from build123d import *

# Parameters (mm, degrees)
SKETCH1_W                       = 28.5
SKETCH1_H                       = 61
SKETCH1_W_2                     = 20.5
SKETCH1_H_2                     = 43
BOSS_EXTRUDE1_DEPTH             = 8
SKETCH2_W                       = 4
SKETCH2_H                       = 52
BOSS_EXTRUDE2_DEPTH             = 55
SKETCH3_W                       = 28.5
SKETCH3_H                       = 12
BOSS_EXTRUDE3_DEPTH             = 4
CUT_EXTRUDE1_DEPTH              = 93.207646104
CUT_EXTRUDE1_DEPTH_BACK         = 93.207646104
SKETCH5_W                       = 15
SKETCH5_H                       = 5.682620757
BOSS_EXTRUDE4_DEPTH             = 20.5
CUT_EXTRUDE2_DEPTH              = 93.207646104
CUT_EXTRUDE2_DEPTH_BACK         = 4
SKETCH7_W                       = 20.5
SKETCH7_H                       = 7
F_3_0MM_DOWEL_HOLE1_D           = 3
F_3_0MM_DOWEL_HOLE1_DEPTH       = 4
F_3_0MM_DOWEL_HOLE1_CSINK_D     = 3.05
F_3_0MM_DOWEL_HOLE1_CSINK_ANGLE = 100
F_3_0MM_DOWEL_HOLE1_TIP         = 0.901290929
SKETCH19_R                      = 2
CUT_EXTRUDE3_DEPTH              = 4
SKETCH21_W                      = 28.5
SKETCH21_H                      = 15
BOSS_EXTRUDE5_DEPTH             = 9
SKETCH24_R                      = 2
CUT_EXTRUDE6_DEPTH              = 14.682620757
CUT_EXTRUDE7_START              = -15
CUT_EXTRUDE7_OUTLINE_W          = 20.5
CUT_EXTRUDE7_OUTLINE_H          = 5.682620757
CUT_EXTRUDE7_DEPTH              = 15
BOSS_EXTRUDE6_DEPTH             = 20.5
SKETCH27_W                      = 28.5
SKETCH27_H                      = 12
BOSS_EXTRUDE7_DEPTH             = 3
SKETCH28_W                      = 20.5
SKETCH28_H                      = 5
CUT_EXTRUDE8_DEPTH              = 15
CUT_EXTRUDE9_START              = -28.5
SKETCH29_R                      = 1.5
CUT_EXTRUDE9_DEPTH              = 28.5


# Read off the part's stored shape, not the designer's step: Cut-Extrude7
with BuildPart() as part:
    # Sketch1 → Boss-Extrude1 (new body)
    with BuildSketch(Plane.XY):
        with Locations((14.25, -30.5)):
            Rectangle(SKETCH1_W, SKETCH1_H)
        with Locations((14.25, -30.5)):
            Rectangle(SKETCH1_W_2, SKETCH1_H_2, mode=Mode.SUBTRACT)
    extrude(amount=BOSS_EXTRUDE1_DEPTH)

    # Sketch2 → Boss-Extrude2 (add)
    with BuildSketch(Plane.XY.offset(8)):
        with Locations((2, -35)):
            Rectangle(SKETCH2_W, SKETCH2_H)
        with Locations((26.5, -35)):
            Rectangle(SKETCH2_W, SKETCH2_H)
    extrude(amount=BOSS_EXTRUDE2_DEPTH)

    # Sketch3 → Boss-Extrude3 (add)
    with BuildSketch(Plane.XZ.offset(61)):
        with Locations((14.25, 57)):
            Rectangle(SKETCH3_W, SKETCH3_H)
        with Locations((14.25, 29)):
            Rectangle(SKETCH3_W, SKETCH3_H)
    extrude(amount=-BOSS_EXTRUDE3_DEPTH)

    # Sketch4 → Cut-Extrude1 (cut, two sides: drawn at the far end of the back side and taken through both)
    with BuildSketch(Plane(origin=(28.5, 0, 0), x_dir=(0, 0, -1), z_dir=(1, 0, 0)).offset(-CUT_EXTRUDE1_DEPTH_BACK)):
        Polygon((-54.327023097, -40.788512694), (-54.327023097, -14.682620757), (-20.327023097, -14.682620757), align=None)
        Polygon((-50.672976903, -45.547498554), (-16.672976903, -45.547498554), (-16.672976903, -19.441606616), align=None)
    extrude(amount=CUT_EXTRUDE1_DEPTH + CUT_EXTRUDE1_DEPTH_BACK, mode=Mode.SUBTRACT)

    # Sketch5 → Boss-Extrude4 (add)
    with BuildSketch(Plane(origin=(4, 0, 0), x_dir=(0, 0, -1), z_dir=(1, 0, 0))):
        with Locations((-30.827023097, -11.841310379)):
            Rectangle(SKETCH5_W, SKETCH5_H)
    extrude(amount=BOSS_EXTRUDE4_DEPTH)

    # Sketch7 → Cut-Extrude2 (cut, two sides: drawn at the far end of the back side and taken through both)
    with BuildSketch(Plane(origin=(0, 0, 0), x_dir=(-1, 0, 0), z_dir=(0, 0, -1)).offset(-CUT_EXTRUDE2_DEPTH_BACK)):
        with Locations((-14.25, -5.5)):
            Rectangle(SKETCH7_W, SKETCH7_H)
        with Locations((-14.25, -55.5)):
            Rectangle(SKETCH7_W, SKETCH7_H)
    extrude(amount=CUT_EXTRUDE2_DEPTH + CUT_EXTRUDE2_DEPTH_BACK, mode=Mode.SUBTRACT)

    # Ø3.0mm Dowel Hole1
    with Locations(Plane(origin=(0, 0, 4), x_dir=(-1, 0, 0), z_dir=(0, 0, -1))):
        with Locations((-19.25, -55), (-9.25, -55), (-19.25, -6), (-9.25, -6)):
            CounterSinkHole(F_3_0MM_DOWEL_HOLE1_D / 2, F_3_0MM_DOWEL_HOLE1_CSINK_D / 2, depth=F_3_0MM_DOWEL_HOLE1_DEPTH, counter_sink_angle=F_3_0MM_DOWEL_HOLE1_CSINK_ANGLE)
            with Locations((0, 0, -(F_3_0MM_DOWEL_HOLE1_DEPTH + F_3_0MM_DOWEL_HOLE1_TIP / 2))):  # 118° drill point
                Cone(0, F_3_0MM_DOWEL_HOLE1_D / 2, F_3_0MM_DOWEL_HOLE1_TIP, mode=Mode.SUBTRACT)

    # Sketch19 → Cut-Extrude3 (cut)
    with BuildSketch(Plane.XZ.offset(61)):
        with Locations(Location((9.25, 57, 0), (0, 0, 270))):
            Circle(SKETCH19_R)
        with Locations(Location((19.25, 57, 0), (0, 0, 270))):
            Circle(SKETCH19_R)
        with Locations(Location((9.25, 29, 0), (0, 0, 270))):
            Circle(SKETCH19_R)
        with Locations(Location((19.25, 29, 0), (0, 0, 270))):
            Circle(SKETCH19_R)
    extrude(amount=-CUT_EXTRUDE3_DEPTH, mode=Mode.SUBTRACT)

    # Sketch21 → Boss-Extrude5 (add)
    with BuildSketch(Plane(origin=(0, -9, 0), x_dir=(1, 0, 0), z_dir=(0, 1, 0))):
        with Locations((14.25, -40.5)):
            Rectangle(SKETCH21_W, SKETCH21_H)
    extrude(amount=BOSS_EXTRUDE5_DEPTH)

    # Sketch24 → Cut-Extrude6 (cut)
    with BuildSketch(Plane(origin=(0, 0, 0), x_dir=(1, 0, 0), z_dir=(0, 1, 0))):
        with Locations(Location((9.25, -40.5, 0), (0, 0, 180))):
            Circle(SKETCH24_R)
        with Locations(Location((19.25, -40.5, 0), (0, 0, 180))):
            Circle(SKETCH24_R)
    extrude(amount=-CUT_EXTRUDE6_DEPTH, mode=Mode.SUBTRACT)

    # Cut-Extrude7 outline → Cut-Extrude7 (cut)
    with BuildSketch(Plane.XY.offset(38.327023097).offset(CUT_EXTRUDE7_START)):
        with Locations((14.25, -11.841310379)):
            Rectangle(CUT_EXTRUDE7_OUTLINE_W, CUT_EXTRUDE7_OUTLINE_H)
    extrude(amount=CUT_EXTRUDE7_DEPTH, mode=Mode.SUBTRACT)

    # Sketch26 → Boss-Extrude6 (add)
    with BuildSketch(Plane(origin=(4, 0, 0), x_dir=(0, 0, -1), z_dir=(1, 0, 0))):
        Polygon((-46.276957579, -42.172145453), (-49.931003773, -37.413159593), (-35.654046194, -26.451021012), (-32, -31.210006872), align=None)
    extrude(amount=BOSS_EXTRUDE6_DEPTH)

    # Sketch27 → Boss-Extrude7 (add)
    with BuildSketch(Plane.XY.offset(63)):
        with Locations((14.25, -27)):
            Rectangle(SKETCH27_W, SKETCH27_H)
    extrude(amount=BOSS_EXTRUDE7_DEPTH)

    # Sketch28 → Cut-Extrude8 (cut)
    with BuildSketch(Plane.XY.offset(48)):
        with Locations((14.25, -6.5)):
            Rectangle(SKETCH28_W, SKETCH28_H)
    extrude(amount=-CUT_EXTRUDE8_DEPTH, mode=Mode.SUBTRACT)

    # Sketch29 → Cut-Extrude9 (cut)
    with BuildSketch(Plane(origin=(28.5, 0, 0), x_dir=(0, 0, -1), z_dir=(1, 0, 0)).offset(CUT_EXTRUDE9_START)):
        with Locations(Location((-58.663511548, -15, 0), (0, 0, 90))):
            Circle(SKETCH29_R)
    extrude(amount=CUT_EXTRUDE9_DEPTH, mode=Mode.SUBTRACT)


solid = part.part
Could you check a few things on this model? Use its own coordinates, in mm. A direction names the side the tool comes from. Give positions to 0.01 mm unless a question says otherwise; leave off trailing zeros. Write each loop counter-clockwise with the first axis right and the second up, starting at its lowest first coordinate (ties: lowest second). Pieces come first, ordered by that corner, then holes. Notation, with made-up numbers: (-34.75, 25) - (21.25, 25) arc R19 ccw to (21.25, 46) - close; hole circle Ø7 at (64, -31). An arc over 180 degrees is marked (long way). Use CSV: the item, a comma, the result in double quotes. Start each with the question number.
Item 1: I want a section at A-A, the plane z = 52. Please give me the cut outline in (x, y).
Item 2: For faces 1 (the face through (2, -33, 16.673)), 2 (the face through (19.684, -1.972, 38.548)), 3 (the face through (2, -15, 63)), 4 (the face through (14, -33, 64)), which set-ups out of +Z, -Z, +X, -X, +Y, -Y let a thin tool reach every point of the face, with its end or its side?
Item 3: I'm going to push flat-ended pins straight in: pin 1 (5 mm diameter, centred on x = 9.25, y = -55, fed in from +Z); pin 2 (1.2 mm diameter, centred on x = 27, z = 52.5, fed in from +Y); pin 3 (7 mm diameter, centred on x = 15.5, y = -6, fed in from +Z). Where does each tip first touch, or does it pass through?
Item 4: I want a section at C-C, the plane y = -35. Please give me the cut outline in (x, z), then the cut area to 3 significant figures.
Item 5: If we mould it in two halves opening along Z, with no side actions, what happens to faces 5 (the face through (14, -5, 4)), 6 (the face through (14, -4, 8)), 7 (the face through (14, -3, 33)), 8 (the face through (14, -3, 48))? For each: pulls with the +Z half, pulls with the -Z half, needs draft (parallel to the pull), parting line crosses it, or undercut.
Item 6: If I drill on line 1 along X through (y, z) = (-55, 5.7); line 2 along Z through (x, y) = (1.3, -15); line 3 along X through (y, z) = (-60, 57), over which ranges is the centre line in solid material (lowest first)?
Item 7: I want a section at B-B, the plane x = 19.25. Give the number of separate pieces and of enclosed holes in the cut face, then the cut area to 3 significant figures.
Findings:
1,outline,"(0, -61) - (28.5, -61) - (28.5, -39) - (24.5, -39) - (24.5, -57) - (4, -57) - (4, -39) - (0, -39) - close; (0, -14.68) - (4, -14.68) - (4, -9) - (0, -9) - close; (24.5, -14.68) - (28.5, -14.68) - (28.5, -9) - (24.5, -9) - close"
2,face 1,"+X, -X"
2,face 2,"+Y"
2,face 3,"+Z, +X, -X, +Y"
2,face 4,"+Z, +X, -X, -Y"
3,pin 1,"stops at z = 63"
3,pin 2,"stops at y = -9"
3,pin 3,"stops at z = 48"
4,outline,"(0, 0) - (4, 0) - (4, 16.67) - (0, 16.67) - close; (0, 36.94) - (28.5, 36.94) - (28.5, 46.79) - (0, 46.79) - close; (0, 54.33) - (4, 54.33) - (4, 63) - (0, 63) - close; (24.5, 0) - (28.5, 0) - (28.5, 16.67) - (24.5, 16.67) - close; (24.5, 54.33) - (28.5, 54.33) - (28.5, 63) - (24.5, 63) - close"
4,area,"484 mm2"
5,face 5,"pulls with the -Z half"
5,face 6,"undercut"
5,face 7,"undercut"
5,face 8,"pulls with the +Z half"
6,line 1,"x = 0 to 7.75, 10.75 to 17.75, 20.75 to 28.5"
6,line 2,"z = 0 to 20.74, 54.33 to 57.16, 60.16 to 63"
6,line 3,"x = 0 to 7.25, 11.25 to 17.25, 21.25 to 28.5"
7,separate pieces,"12"
7,enclosed holes,"0"
7,area,"316 mm2"
